Read the model definition and answer for the solid it produces. Units are mm, in the model's axes. Give positions to 0.01 mm unless a question says otherwise; leave off trailing zeros. Loops run counter-clockwise (first coordinate to the right, second up) from the corner with the lowest first, then second, coordinate; pieces in that order, holes last. Notation, with made-up numbers: (27.25, -21.5) -> (77.25, -21.5) arc R28 ccw to (77.25, 16.5) -> close; hole circle Ø7 at (77, 39.5). An arc over 180 degrees is marked (long way). One line per item, written item: value. Start each with the question number.
from build123d import *

# Parameters (mm, degrees)
BOSS_EXTRUDE1_DEPTH = 1.5875
SKETCH3_R           = 1
CUT_EXTRUDE2_DEPTH  = 3.175


with BuildPart() as part:
    # Sketch1 → Boss-Extrude1 (new, symmetric)
    with BuildSketch(Plane.XY.offset(264.790013628)):
        with BuildLine():
            Line((33.800017398, -5.067355161), (33.800017398, 13.955458653))
            ThreePointArc((33.800017398, 13.955458653), (0, 33.800390955), (-33.800017398, 13.955458653))
            Line((-33.800017398, 13.955458653), (-33.800017398, -5.067355161))
            add(Edge.make_bspline(
                [(-33.800017398, -5.067355161), (-33.694935477, -5.172128399), (-33.608288469, -5.290004795), (-33.472323961, -5.552290639), (-33.425425948, -5.692889236), (-33.399533932, -5.838970624)],
                knots=[0, 0, 0, 0, 0.5, 0.5, 1, 1, 1, 1], degree=3))
            add(Edge.make_bspline(
                [(-33.399533932, -5.838970624), (-33.052253285, -7.798309693), (-32.28122422, -10.647467269), (-31.145731134, -13.365691593), (-30.518165219, -14.703313718), (-30.29902031, -15.145610982), (-29.840887044, -16.023076775), (-29.601228036, -16.459250859), (-28.359208449, -18.607369492), (-27.22981433, -20.215826589), (-25.018856718, -22.840568094), (-23.995930567, -23.90437348), (-22.532682873, -25.242268373), (-22.158108065, -25.570446836), (-20.260791979, -27.161701153), (-18.652171115, -28.2877371), (-16.102983861, -29.756171424), (-15.230549353, -30.208885919), (-13.44029889, -31.040835285), (-12.518244043, -31.421602723), (-9.730335127, -32.436850643), (-7.835048114, -32.947048229), (-4.936180491, -33.458234156), (-3.960569712, -33.586283528), (-1.990568761, -33.757071458), (-0.994552943, -33.799592721), (7.014e-06, -33.799609106)],
                knots=[0, 0, 0, 0, 0.125, 0.1875, 0.1875, 0.21875, 0.21875, 0.25, 0.25, 0.375, 0.375, 0.46875, 0.46875, 0.5, 0.5, 0.625, 0.625, 0.6875, 0.6875, 0.75, 0.75, 0.875, 0.875, 0.9375, 0.9375, 1, 1, 1, 1], degree=3))
            add(Edge.make_bspline(
                [(7.014e-06, -33.799609106), (1.987875992, -33.799575566), (3.94703991, -33.631115611), (6.842232548, -33.122877847), (8.278942061, -32.804880827), (9.699244221, -32.390613968), (10.642458673, -32.092998308), (11.113286404, -31.933080905), (13.444877358, -31.084762204), (15.228063078, -30.258192227), (18.202438097, -28.548252781), (19.430049544, -27.730513432), (21.002878368, -26.524895287), (21.391487804, -26.213219806), (23.290603811, -24.621354585), (24.683841541, -23.235802325), (26.897817983, -20.611786452), (27.77410108, -19.422700527), (28.842940769, -17.748765821), (29.101464741, -17.323406575), (30.340761198, -15.181007143), (31.176382916, -13.403126413), (32.193288505, -10.639212594), (32.492355328, -9.701528607), (33.008528869, -7.792516567), (33.225825771, -6.819022893), (33.399533932, -5.838970624)],
                knots=[0, 0, 0, 0, 0.125, 0.125, 0.1875, 0.21875, 0.21875, 0.25, 0.25, 0.375, 0.375, 0.46875, 0.46875, 0.5, 0.5, 0.625, 0.625, 0.71875, 0.71875, 0.75, 0.75, 0.875, 0.875, 0.9375, 0.9375, 1, 1, 1, 1], degree=3))
            add(Edge.make_bspline(
                [(33.399533932, -5.838970624), (33.425419923, -5.692923228), (33.471627634, -5.554074987), (33.607200861, -5.29166755), (33.694927142, -5.172136709), (33.800017398, -5.067355161)],
                knots=[0, 0, 0, 0, 0.5, 0.5, 1, 1, 1, 1], degree=3))
        make_face()
    extrude(amount=BOSS_EXTRUDE1_DEPTH, both=True)

    # Sketch3 → Cut-Extrude2 (cut)
    with BuildSketch(Plane.XY.offset(266.377513628)):
        with Locations((-31.216064399, -8.164436653)):
            Circle(SKETCH3_R)
        with Locations((32.009302375, -5.358989516)):
            Circle(SKETCH3_R)
    extrude(amount=-CUT_EXTRUDE2_DEPTH, mode=Mode.SUBTRACT)


solid = part.part
Item 1: Section C-C, the plane y = 20 is taken. Determine the outline of the cut face in (x, z), plus the area to 3 significant figures.
Item 2: Consider L1, parallel to Y at x = -0.5, z = 264; L2, parallel to Y at x = -29, z = 265.2; L3, parallel to X at y = -10.5, z = 266. Determine where each line is inside the solid, lowest interval first. Write a range as [from, to].
Item 3: Determine the mould class of faces 1 (the flat face through (0, 0, 266.378)), 2 (the cylindrical face through (0.575, 33.796, 264.812)), 3 (the flat face through (33.8, 4, 265)), 4 (the cylindrical face through (-32.215, -8.12, 264.812)) for opening direction X: pulls with the +X half, pulls with the -X half, needs draft (parallel to the pull), parting line crosses it, or undercut.
Item 4: Section A-A, the plane z = 264 is taken. State how many separate pieces and enclosed holes the cut face has, plus the area to 3 significant figures.
Item 5: Section B-B, the plane y = 27 is taken. Determine the outline of the cut face in (x, z).
Item 6: Flat-ended cylindrical pins translate along their axes: pin 1 (2.5 mm diameter, centred on x = 32.01, y = -5.36, fed in from +Z); pin 2 (1 mm diameter, centred on x = 8.5, z = 265, fed in from +Y). Find the tip coordinate at first contact, or state that the pin passes through.
Computed values:
1. outline: (-29.63, 263.2) -> (29.63, 263.2) -> (29.63, 266.38) -> (-29.63, 266.38) -> close
1. area: 188 mm²
2. L1: [-33.8, 33.8]
2. L2: [-17.49, 20.73]
2. L3: [-32.22, 32.22]
3. face 1: needs draft
3. face 2: parting line crosses it
3. face 3: pulls with the +X half
3. face 4: undercut
4. separate pieces: 1
4. enclosed holes: 2
4. area: 3,690 mm²
5. outline: (-21.91, 263.2) -> (21.91, 263.2) -> (21.91, 266.38) -> (-21.91, 266.38) -> close
6. pin 1: z = 266.38
6. pin 2: y = 32.96
